Could you check a few things on this drawing? It's one solid part, dimensions in mm from its lowest x, y, z. A direction names the side the tool comes from. Coordinates: 2 decimals unless noted, no trailing zeros. Order: outer loops, then holes, each group sorted by start corner. A loop starts at its lowest first (then second) coordinate and runs counter-clockwise, first axis right, second up. Notation, with made-up numbers: M 18.5,-25.5 L 57.5,-25.5 A14 cw 57.5,-13.5 Z; hole C -15,11.5 d8. An arc over 180 degrees is marked long. Answer as CSV lines item,"result". Start each with the question number.
1. I need wall thicknesses on line 1 along X through (y, z) = (7.5, 27); line 2 along Z through (x, y) = (49, 4); line 3 along X through (y, z) = (7.75, 20). Which ranges of each line are inside material? Lowest first, please. Write a range as from..to.
2. If we section it at C-C (x = 29): List the corners of the cut face in (y, z) for me, plus the area to 3 significant figures.
3. If we mould it in two halves opening along X, with no side actions, what happens to the marked faces 4, 5, 6 and 7? For each: released by +X, released by -X, zero draft, split by the parting line, or undercut.
4. On a 3-axis mill with a long thin cutter (end or side, diameter ignored), from which of +Z, -Z, +X, -X, +Y, -Y can I reach the whole of each face in a straight line? I mean the marked faces 1, 2 and 3. Say none if no direction works.
5. If we section it at B-B (x = 9): List the corners of the cut face in (y, z) for me.
6. If we section it at A-A (y = 4): List the corners of the cut face in (x, z) for me.
7. Will these pins go through, and if not, where does the flat tip stop? pin 1 (3.5 mm diameter, centred on y = 2, z = 19, fed in from -X); pin 2 (5 mm diameter, centred on y = 4, z = 21.5, fed in from +X); pin 3 (2 mm diameter, centred on x = 54, y = 8, fed in from +Z); pin 4 (10 mm diameter, centred on x = 30.5, z = 33, fed in from -Y).
8. If we section it at D-D (y = 8.25): List the corners of the cut face in (x, z) for me, plus the area to 3 significant figures.
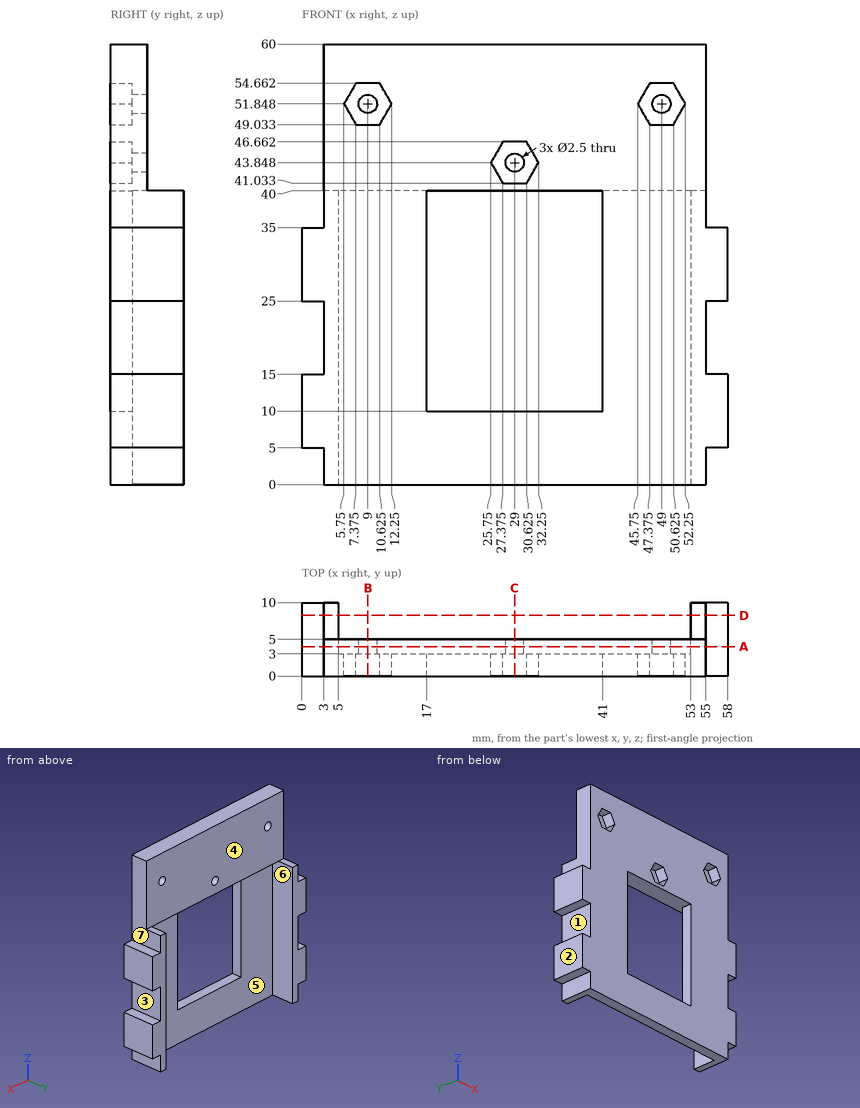
Solved:
1,line 1,"0..5, 53..58"
1,line 2,"40..50.6, 53.1..60"
1,line 3,"3..5, 53..55"
2,outline,"M 0,0 L 3,0 L 3,10 L 0,10 Z; M 0,40 L 5,40 L 5,42.6 L 3,42.6 L 3,41.03 L 0,41.03 Z; M 0,46.66 L 3,46.66 L 3,45.1 L 5,45.1 L 5,60 L 0,60 Z"
2,area,"108 mm²"
3,face 4,"zero draft"
3,face 5,"undercut"
3,face 6,"undercut"
3,face 7,"released by +X"
4,face 1,"-X, +Y, -Y"
4,face 2,"+Z, -Z, -X, +Y, -Y"
4,face 3,"+X, +Y, -Y"
5,outline,"M 0,0 L 3,0 L 3,40 L 5,40 L 5,50.6 L 3,50.6 L 3,49.03 L 0,49.03 Z; M 0,54.66 L 3,54.66 L 3,53.1 L 5,53.1 L 5,60 L 0,60 Z"
6,outline,"M 0,5 L 3,5 L 3,0 L 5,0 L 5,40 L 53,40 L 53,0 L 55,0 L 55,5 L 58,5 L 58,15 L 55,15 L 55,25 L 58,25 L 58,35 L 55,35 L 55,60 L 3,60 L 3,35 L 0,35 L 0,25 L 3,25 L 3,15 L 0,15 Z; hole C 9,51.85 d2.5; hole C 29,43.85 d2.5; hole C 49,51.85 d2.5"
7,pin 1,"x = 3"
7,pin 2,"x = 55"
7,pin 3,"z = 40"
7,pin 4,"through"
8,outline,"M 0,5 L 3,5 L 3,0 L 5,0 L 5,40 L 3,40 L 3,35 L 0,35 L 0,25 L 3,25 L 3,15 L 0,15 Z; M 53,0 L 55,0 L 55,5 L 58,5 L 58,15 L 55,15 L 55,25 L 58,25 L 58,35 L 55,35 L 55,40 L 53,40 Z"
8,area,"280 mm²"
